Source: CAD feature listing. Evaluate the final solid. Frame: model axes, mm. Give positions to 0.01 mm unless a question says otherwise; leave off trailing zeros. Write each loop counter-clockwise with the first axis right and the second up, starting at its lowest first coordinate (ties: lowest second). Pieces come first, ordered by that corner, then holes. Notation, with made-up numbers: (31, 75) -> (84, 75) arc R10 cw to (84, 90) -> close; hole circle Ø3 at (81, -38). An arc over 180 degrees is marked (long way). Answer as a JSON object with one key per item and string values. Group by question number.
Item 1: Ray query, probe 1 along X at (y, z) = (75, -5); probe 2 along X at (y, z) = (39.5, 3.5); probe 3 along Z at (x, y) = (-11.5, 52.5). Return the intervals inside material, ascending. Write a range as from..to.
Item 2: Pull-direction query (X, two-part tool) for faces 1 (the face through (0, 89, -29.837)), 2 (the face through (13.423, 88.782, -2.857)), 3 (the face through (-14.293, 91.26, 8.254)); classes: pulls with the +X half, pulls with the -X half, needs draft (parallel to the pull), parting line crosses it, or undercut.
Item 3: Section query B-B on y = 120.5. Return the cut outline in (x, z).
Item 4: First-contact query: pin 1 Ø10 at (x, y) = (-12.5, 116.5) entering from +Z; pin 2 Ø5 at (x, z) = (-8, -15.5) entering from -Y; pin 3 Ø10 at (x, z) = (4.5, -8) entering from -Y; pin 4 Ø2 at (x, y) = (-7, 120) entering from +Z. Flat tips, straight axial feed; report the tip coordinate or a pass-through.
Item 5: Section query A-A on x = 0. Return the cut outline in (y, z), plus the area to 3 significant figures.
from build123d import *

# Parameters (mm, degrees)
SKETCH1_R           = 13.75
BOSS_EXTRUDE1_DEPTH = 180
FILLET1_R           = 13
FILLET2_R           = 3


with BuildPart() as part:
    # Sketch1 → Boss-Extrude1 (new body)
    with BuildSketch(Plane(origin=(0, 0, 0), x_dir=(1, 0, 0), z_dir=(0, 1, 0))):
        Polygon((0, 29.837240524), (-18, 29.837240524), (-18, -12.162759476), (18, -12.162759476), (18, 29.837240524), align=None)
        with Locations(Location((0, 5.837240524, 0), (0, 0, 90))):
            Circle(SKETCH1_R, mode=Mode.SUBTRACT)
    extrude(amount=BOSS_EXTRUDE1_DEPTH)

    # Fillet1
    fillet1_edges = [part.edges().sort_by_distance(p)[0] for p in [
        (18, 90, 12.162759476),
        (-18, 90, 12.162759476),
    ]]
    fillet(fillet1_edges, radius=FILLET1_R)

    # Fillet2
    fillet2_edges = [part.edges().sort_by_distance(p)[0] for p in [
        (0, 0, 7.912759476),
        (0, 180, 7.912759476),
    ]]
    fillet(fillet2_edges, radius=FILLET2_R)


solid = part.part
Worked answers:
{
 "1": {"probe 1": "-18..-13.72, 13.72..18", "probe 2": "-17.26..-10.09, 10.09..17.26", "probe 3": "-29.84..-13.37, 1.7..10.42"},
 "2": {"face 1": "needs draft", "face 2": "undercut", "face 3": "pulls with the -X half"},
 "3": {"outline": "(-18, -29.84) -> (18, -29.84) -> (18, -0.84) arc R13 ccw to (5, 12.16) -> (-5, 12.16) arc R13 ccw to (-18, -0.84) -> close; hole circle Ø27.5 at (0, -5.84)"},
 "4": {"pin 1": "z = 11.92", "pin 2": "y = 0.53", "pin 3": "through", "pin 4": "z = 12.12"},
 "5": {"outline": "(0, -29.84) -> (180, -29.84) -> (180, -22.59) arc R3 ccw to (177, -19.59) -> (3, -19.59) arc R3 ccw to (0, -22.59) -> close; (0, 10.91) arc R3 ccw to (3, 7.91) -> (177, 7.91) arc R3 ccw to (180, 10.91) -> (180, 12.16) -> (0, 12.16) -> close", "area": "2,600 mm^2"}
}
